For this review, take the finished solid that the model builds, in its own axes (mm). A direction names the side the tool comes from. Give positions to 0.01 mm unless a question says otherwise; leave off trailing zeros. Loops run counter-clockwise (first coordinate to the right, second up) from the corner with the lowest first, then second, coordinate; pieces in that order, holes last.
```python
from build123d import *

# Parameters (mm, degrees)
SKETCH_1_R          = 75
EXTRUDE_1_DEPTH     = 26
SKETCH_3_R          = 67.5
CUT_EXTRUDE_2_DEPTH = 13
SKETCH_4_R          = 4.5
CUT_EXTRUDE_3_DEPTH = 110.206226929
SKETCH_5_R          = 25
EXTRUDE_2_DEPTH     = 5
SKETCH_8_R          = 17.5
EXTRUDE_4_DEPTH     = 23


with BuildPart() as part:
    # 草图1 → 拉伸1 (new body)
    with BuildSketch(Plane.XY):
        with Locations(Location((0, 0, 0), (0, 0, 180))):
            Circle(SKETCH_1_R)
    extrude(amount=EXTRUDE_1_DEPTH)

    # 草图3 → 切除-拉伸2 (cut)
    with BuildSketch(Plane.XY.offset(26)):
        Circle(SKETCH_3_R)
    extrude(amount=-CUT_EXTRUDE_2_DEPTH, mode=Mode.SUBTRACT)

    # 草图4 → 切除-拉伸3 (cut, through all)
    with BuildSketch(Plane(origin=(0, 0, 0), x_dir=(-1, 0, 0), z_dir=(0, 0, -1))):
        with Locations((0, 60)):
            Circle(SKETCH_4_R)
        with Locations((51.961524227, 30)):
            Circle(SKETCH_4_R)
        with Locations((51.961524227, -30)):
            Circle(SKETCH_4_R)
        with Locations((0, -60)):
            Circle(SKETCH_4_R)
        with Locations((-51.961524227, -30)):
            Circle(SKETCH_4_R)
        with Locations((-51.961524227, 30)):
            Circle(SKETCH_4_R)
    extrude(amount=-CUT_EXTRUDE_3_DEPTH, mode=Mode.SUBTRACT)

    # 草图5 → 拉伸2 (add)
    with BuildSketch(Plane(origin=(0, 0, 0), x_dir=(-1, 0, 0), z_dir=(0, 0, -1))):
        with Locations(Location((0, 0, 0), (0, 0, 180))):
            Circle(SKETCH_5_R)
    extrude(amount=EXTRUDE_2_DEPTH)

    # 草图8 → 拉伸4 (add)
    with BuildSketch(Plane(origin=(0, 0, -5), x_dir=(-1, 0, 0), z_dir=(0, 0, -1))):
        Circle(SKETCH_8_R)
    extrude(amount=EXTRUDE_4_DEPTH)


solid = part.part
```
Q1. Consider section B-B on x = 0. Give the boundary of the cut face in (y, z).
Answers:
outline: (-75, 0) - (-64.5, 0) - (-64.5, 13) - (-67.5, 13) - (-67.5, 26) - (-75, 26) - close; (-55.5, 0) - (-25, 0) - (-25, -5) - (-17.5, -5) - (-17.5, -28) - (17.5, -28) - (17.5, -5) - (25, -5) - (25, 0) - (55.5, 0) - (55.5, 13) - (-55.5, 13) - close; (64.5, 0) - (75, 0) - (75, 26) - (67.5, 26) - (67.5, 13) - (64.5, 13) - close
Q2. Machinability: for faces 5 (the cylindrical face through (13.887, -10.648, -16.339)), 6 (the cylindrical face through (0.98, 55.61, 6.41)), 7 (the cylindrical face through (-53.57, -41.07, 19.59)), which of the approach directions +Z, -Z, +X, -X, +Y, -Y give a long, thin tool a straight path to every point of the face, cutting with its end or side? Answer none if there is none.
Answers:
face 5: -Z
face 6: +Z, -Z
face 7: +Z
Q3. Consider section C-C on y = 0. Give the boundary of the cut face in (x, z), plus the area to 3 significant figures.
Answers:
outline: (-75, 0) - (-25, 0) - (-25, -5) - (-17.5, -5) - (-17.5, -28) - (17.5, -28) - (17.5, -5) - (25, -5) - (25, 0) - (75, 0) - (75, 26) - (67.5, 26) - (67.5, 13) - (-67.5, 13) - (-67.5, 26) - (-75, 26) - close
area: 3,200 mm2
Q4. Consider section D-D on y = 60. Give the boundary of the cut face in (x, z), plus the area to 3 significant figures.
Answers:
outline: (-45, 0) - (-4.5, 0) - (-4.5, 13) - (-30.92, 13) - (-30.92, 26) - (-45, 26) - close; (4.5, 0) - (45, 0) - (45, 26) - (30.92, 26) - (30.92, 13) - (4.5, 13) - close
area: 1,420 mm2
Q5. For pin 1 Ø8 at (x, y) = (51.96, -30) entering from -Z; pin 2 Ø6 at (x, z) = (-40, 16.5) entering from -Y; pin 3 Ø1 at (x, y) = (-32, 37) entering from +Z; pin 4 Ø6 at (y, z) = (-3, -9) entering from -X, all flat-tipped, find the tip position at first contact; note any pin that passes through.
Answers:
pin 1: passes through
pin 2: stops at y = -65.24
pin 3: stops at z = 13
pin 4: stops at x = -17.5
Q6. For probe 1 along Y at (x, z) = (0, 8); probe 2 along Y at (x, z) = (-50, 9); probe 3 along Y at (x, z) = (0, 19), list the stretches that pass through material, from the lowest coordinate up.
Answers:
probe 1: y = -75 to -64.5, -55.5 to 55.5, 64.5 to 75
probe 2: y = -55.9 to -34.05, -25.95 to 25.95, 34.05 to 55.9
probe 3: y = -75 to -67.5, 67.5 to 75
Q7. Mouldability with a two-part tool opening along Y and no side actions: class faces 1 (the flat face through (-17, 5, -5)), 2 (the cylindrical face through (-34.608, 66.538, 12.818)), 3 (the cylindrical face through (-56.12, 28.28, 6.41)), 4 (the cylindrical face through (56.457, -29.802, 6.409)) as +Y half, -Y half, draft (parallel to the pull), parting line (faces both ways), or undercut.
Answers:
face 1: draft
face 2: parting line
face 3: undercut
face 4: undercut
Q8. Consider section A-A on z = 3.5. Give the boundary of the cut face in (x, y).
Answers:
outline: circle Ø150 at (0, 0); hole circle Ø9 at (-51.96, -30); hole circle Ø9 at (-51.96, 30); hole circle Ø9 at (0, -60); hole circle Ø9 at (0, 60); hole circle Ø9 at (51.96, -30); hole circle Ø9 at (51.96, 30)
